The drawing under review shows one solid part. Ordinate dimensions are in mm from its lowest x, y, z. A direction names the side the tool comes from. Coordinates: 2 decimals unless noted, no trailing zeros. Order: outer loops, then holes, each group sorted by start corner. A loop starts at its lowest first (then second) coordinate and runs counter-clockwise, first axis right, second up. Notation, with made-up numbers: (51, 50) - (58, 50) arc R24 ccw to (58, 79) - close; hole circle Ø11 at (8.5, 23.5). An arc over 180 degrees is marked (long way). Answer in a Markdown table with one row per item.
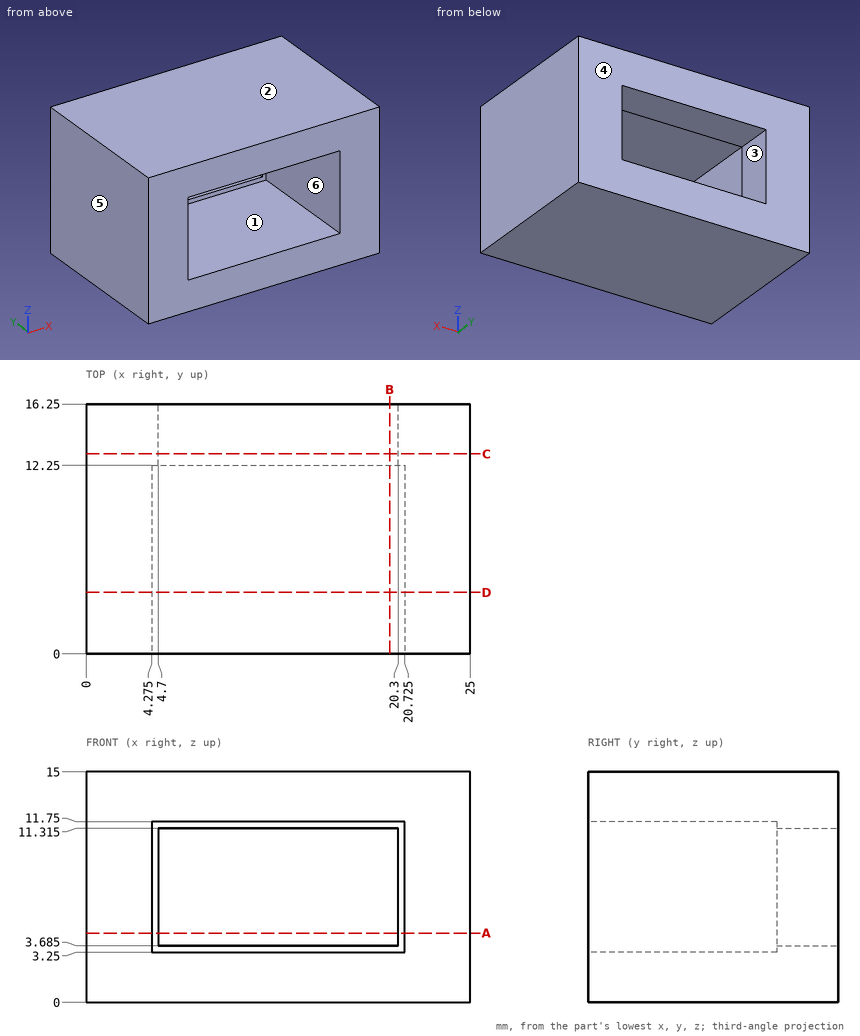
Item 1: Mouldability with a two-part tool opening along X and no side actions: class the marked faces 4, 5 and 6 as +X half, -X half, draft (parallel to the pull), parting line (faces both ways), or undercut.
Check values:
| item | result |
|---|---|
| face 4 | draft |
| face 5 | -X half |
| face 6 | undercut |
Item 2: Tool access review of the marked faces 1, 2 and 3: name each direction out of +Z, -Z, +X, -X, +Y, -Y from which nothing blocks a thin tool from reaching the whole face with its end or side.
Check values:
| item | result |
|---|---|
| face 1 | -Y |
| face 2 | +Z, +X, -X, +Y, -Y |
| face 3 | +Y, -Y |
Item 3: We need section D-D, the plane y = 4. Write out the cut boundary in (x, z) (3 decimals).
Check values:
| item | result |
|---|---|
| outline | (0, 0) - (25, 0) - (25, 15) - (0, 15) - close; hole (4.275, 3.25) - (20.725, 3.25) - (20.725, 11.75) - (4.275, 11.75) - close |
Item 4: We need section C-C, the plane y = 13. Write out the cut boundary in (x, z) (3 decimals), then the cut area to 3 significant figures.
Check values:
| item | result |
|---|---|
| outline | (0, 0) - (25, 0) - (25, 15) - (0, 15) - close; hole (4.7, 3.685) - (20.3, 3.685) - (20.3, 11.315) - (4.7, 11.315) - close |
| area | 256 mm^2 |
Item 5: We need section A-A, the plane z = 4.5. Write out the cut boundary in (x, y) (3 decimals), then the cut area to 3 significant figures.
Check values:
| item | result |
|---|---|
| outline | (0, 0) - (4.275, 0) - (4.275, 12.25) - (4.7, 12.25) - (4.7, 16.25) - (0, 16.25) - close; (20.3, 12.25) - (20.725, 12.25) - (20.725, 0) - (25, 0) - (25, 16.25) - (20.3, 16.25) - close |
| area | 142 mm^2 |
Item 6: We need section B-B, the plane x = 19.75. Write out the cut boundary in (y, z) (3 decimals).
Check values:
| item | result |
|---|---|
| outline | (0, 0) - (16.25, 0) - (16.25, 3.685) - (12.25, 3.685) - (12.25, 3.25) - (0, 3.25) - close; (0, 11.75) - (12.25, 11.75) - (12.25, 11.315) - (16.25, 11.315) - (16.25, 15) - (0, 15) - close |
Item 7: To check wall thickness, follow line 1 (X direction, y = 8.75, z = 6.75) (3 decimals); line 2 (X direction, y = 14.25, z = 5); line 3 (Z direction, x = 6, y = 1.5). State the ranges of each line that lie inside material, in increasing order. Write a range as from..to.
Check values:
| item | result |
|---|---|
| line 1 | 0..4.275, 20.725..25 |
| line 2 | 0..4.7, 20.3..25 |
| line 3 | 0..3.25, 11.75..15 |
